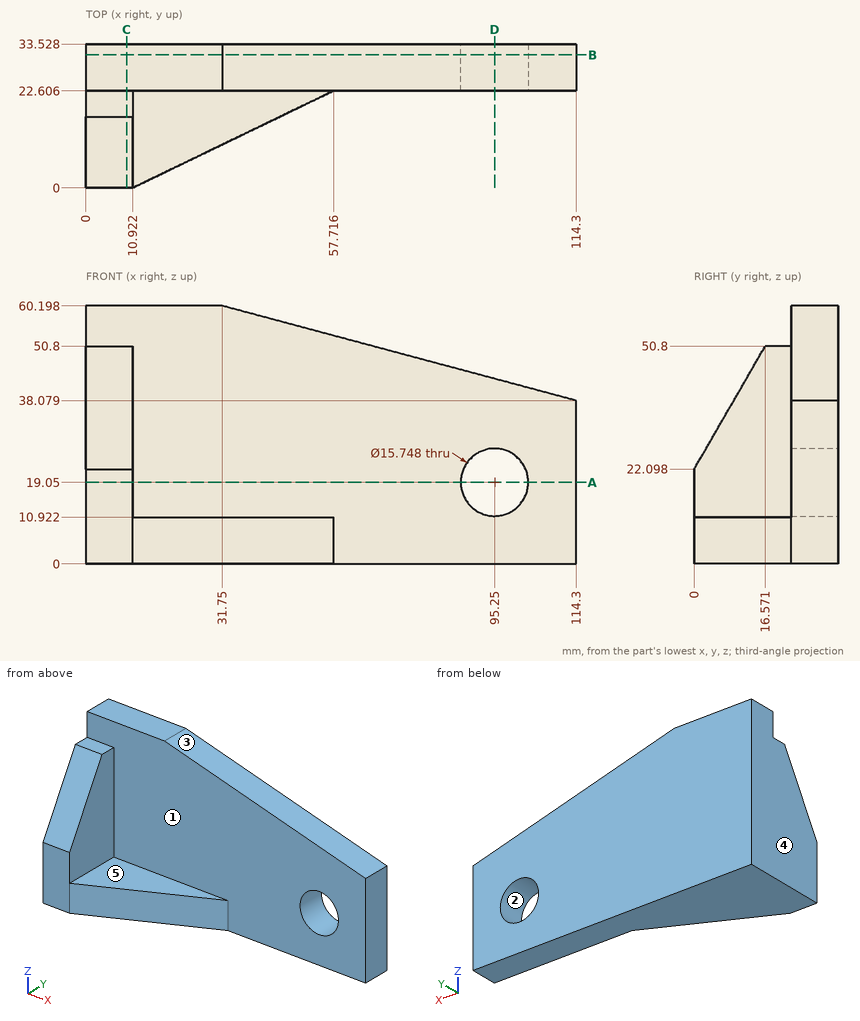
The figure shows three views and two pictorial views of one solid part (mm, origin at its lowest corner). Answer the questions. A direction names the side the tool comes from. Coordinates: 2 decimals unless noted, no trailing zeros. Loops run counter-clockwise (first coordinate to the right, second up) from the corner with the lowest first, then second, coordinate; pieces in that order, holes last. Notation, with made-up numbers: (15.5, 84.25) -> (25.5, 84.25) arc R10 cw to (25.5, 94.25) -> close; hole circle Ø1 at (14, 64.5). An arc over 180 degrees is marked (long way). Use one line per item in the form item = value. Start each with the question number.
Item 1: The part is cut by section C-C on x = 9.5. Determine the outline of the cut face in (y, z), then the cut area to 3 significant figures.
Item 2: The part is cut by section D-D on x = 95.25. Determine the outline of the cut face in (y, z).
Item 3: A tool of negligible diameter and unlimited length cuts with its end or side. For the marked faces 4 and 5, from which of +Z, -Z, +X, -X, +Y, -Y can it reach the whole face along a straight path? Write none if from no direction.
Item 4: Consider L1, parallel to Y at x = 39, z = 33.5; L2, parallel to Z at x = 95, y = 28; L3, parallel to Z at x = 95.25, y = 26.5 (1 decimal). Determine where each line is inside the solid, lowest interval first. Write a range as [from, to].
Item 5: The part is cut by section B-B on y = 31. Determine the outline of the cut face in (x, z).
Item 6: The part is cut by section A-A on z = 19.05. Determine the outline of the cut face in (x, y), then the cut area to 3 significant figures.
Item 7: The mould has two halves that part along Z. Classify the marked faces 1, 2 and 3: released by +Z, released by -Z, zero draft, split by the parting line, or undercut.
Item 8: Flat-ended cylindrical pins translate along their axes: pin 1 Ø7 at (y, z) = (14, 35.5) entering from +X; pin 2 Ø3 at (x, y) = (53, 21) entering from +Z; pin 3 Ø5 at (x, z) = (73, 12.5) entering from -Y. Find the tip coordinate at first contact, or state that the pin passes through.
Answer key:
q1.outline = (0, 0) -> (33.53, 0) -> (33.53, 60.2) -> (22.61, 60.2) -> (22.61, 50.8) -> (16.57, 50.8) -> (0, 22.1) -> close
q1.area = 1,570 mm2
q2.outline = (22.61, 0) -> (33.53, 0) -> (33.53, 11.18) -> (22.61, 11.18) -> close; (22.61, 26.92) -> (33.53, 26.92) -> (33.53, 43.18) -> (22.61, 43.18) -> close
q3.face_4 = +Z, -Z, -X, +Y, -Y
q3.face_5 = +Z, +X, -Y
q4.L1 = [22.61, 33.53]
q4.L2 = [0, 11.18], [26.92, 43.25]
q4.L3 = [0, 11.2], [26.9, 43.2]
q5.outline = (0, 0) -> (114.3, 0) -> (114.3, 38.08) -> (31.75, 60.2) -> (0, 60.2) -> close; hole circle Ø15.75 at (95.25, 19.05)
q6.outline = (0, 0) -> (10.92, 0) -> (10.92, 22.61) -> (87.38, 22.61) -> (87.38, 33.53) -> (0, 33.53) -> close; (103.12, 22.61) -> (114.3, 22.61) -> (114.3, 33.53) -> (103.12, 33.53) -> close
q6.area = 1,320 mm2
q7.face_1 = zero draft
q7.face_2 = undercut
q7.face_3 = released by +Z
q8.pin_1 = 10.92
q8.pin_2 = 10.92
q8.pin_3 = 22.61
